```python
from build123d import *

# Parameters (mm, degrees)
CUT_EXTRUDE_1_DEPTH = 40.276397034
SKETCH_5_W          = 5
SKETCH_5_H          = 6.5
CUT_EXTRUDE_2_DEPTH = 5


with BuildPart() as part:
    # 스케치3 → 로프트1 section 0
    with BuildSketch(Plane.XY):
        with BuildLine():
            Line((-4.446445939, 11.389549668), (4.446445939, 11.389549668))
            Line((4.446445939, 11.389549668), (7.568785652, -1.099809185))
            Line((7.568785652, -1.099809185), (2.355626001, -23.693983454))
            Line((2.355626001, -23.693983454), (-2.355626001, -23.693983454))
            Line((-2.355626001, -23.693983454), (-7.568785652, -1.099809185))
            Line((-7.568785652, -1.099809185), (-4.446445939, 11.389549668))
        make_face()
    # 스케치4 → 로프트1 section 1
    with BuildSketch(Plane.XY.offset(30)):
        with BuildLine():
            Line((-4.342329219, 11.806016546), (4.342329219, 11.806016546))
            Line((4.342329219, 11.806016546), (7.568785652, -1.099809185))
            Line((7.568785652, -1.099809185), (2.240260872, -24.193983454))
            Line((2.240260872, -24.193983454), (-2.240260872, -24.193983454))
            Line((-2.240260872, -24.193983454), (-7.568785652, -1.099809185))
            Line((-7.568785652, -1.099809185), (-4.342329219, 11.806016546))
        make_face()
    loft()

    # 스케치1 → 컷-돌출1 (cut, through all)
    with BuildSketch(Plane.XY):
        Polygon((2.5, 6.806016546), (-2.5, 6.806016546), (-4.5, -1.193983454), (-1.9, -15.193983454), (1.9, -15.193983454), (4.5, -1.193983454), align=None)
    extrude(amount=CUT_EXTRUDE_1_DEPTH, mode=Mode.SUBTRACT)

    # 스케치5 → 컷-돌출2 (cut)
    with BuildSketch(Plane(origin=(0, 0, 0), x_dir=(-1, 0, 0), z_dir=(0, 0, -1))):
        with Locations((0, 10.056016546)):
            Rectangle(SKETCH_5_W, SKETCH_5_H)
    extrude(amount=-CUT_EXTRUDE_2_DEPTH, mode=Mode.SUBTRACT)


solid = part.part
```
Work out the finished part from the listing and answer in its coordinate system (mm). A direction names the side the tool comes from. Round coordinates to 2 decimals unless told otherwise and drop trailing zeros.
Q1. The mould has two halves that part along Y. Classify faces 4 (the flat face through (-4, -6, 0)), 5 (the flat face through (3.5, 2.8, 14.8)): pulls with the +Y half, pulls with the -Y half, needs draft (parallel to the pull), parting line crosses it, or undercut.
Solution:
face 4: needs draft
face 5: undercut
Q2. Find the intervals of material crossed by line 1 along Y through (x, z) = (-1, 25); line 2 along Y through (x, z) = (1.5, 16.5); line 3 along X through (y, z) = (-4.5, 14.5), in increasing order.
Solution:
line 1: y = -24.11 to -15.19, 6.81 to 11.74
line 2: y = -23.97 to -15.19, 6.81 to 11.62
line 3: x = -6.78 to -3.89, 3.89 to 6.78
Q3. A tool of negligible diameter and unlimited length cuts with its end or side. For faces 1 (the flat face through (4, -5, 30)), 2 (the flat face through (-3.218, -8.096, 14.79)), 3 (the flat face through (0, 9, 5)), from which of +Z, -Z, +X, -X, +Y, -Y can it reach the whole face along a straight path? Write none if from no direction.
Solution:
face 1: +Z, +X, -X, +Y, -Y
face 2: +Z, -Z
face 3: -Z, +Y
Q4. Given pin 1 Ø3 at (x, z) = (-3, 7.5) entering from +Y; pin 2 Ø8 at (x, z) = (-5.5, 15.5) entering from -Y; pin 3 Ø5 at (x, y) = (-5, -5) entering from -Z; pin 4 Ø3 at (x, z) = (3.5, 25.5) entering from -Y, each flat-ended and moving along its own axis, determine where each tip first touches the part or whether it passes through.
Solution:
pin 1: stops at y = 11.51
pin 2: stops at y = -23.99
pin 3: stops at z = 0
pin 4: stops at y = -24.13
